```python
from build123d import *

# Parameters (mm, degrees)
BOSS_EXTRUDE1_DEPTH = 4


with BuildPart() as part:
    # Sketch1 → Boss-Extrude1 (new body)
    with BuildSketch(Plane.XY):
        with BuildLine():
            Line((6.07568334, -11), (11.008857545, -11))
            Line((11.008857545, -11), (11.008857545, 0))
            ThreePointArc((11.008857545, 0), (9.544391451, 3.535533906), (6.008857545, 5))
            Line((6.008857545, 5), (-5.92431666, 5))
            Line((-5.92431666, 5), (-5.92431666, -11))
            Line((-5.92431666, -11), (-1.92431666, -11))
            Line((-1.92431666, -11), (-1.92431666, -15))
            Line((-1.92431666, -15), (6.07568334, -15))
            Line((6.07568334, -15), (6.07568334, -11))
        make_face()
    extrude(amount=BOSS_EXTRUDE1_DEPTH)


solid = part.part
```
The model under review builds one solid part; all positions refer to its coordinate system, in mm. A direction names the side the tool comes from. Coordinates: 2 decimals unless noted, no trailing zeros. Write each loop counter-clockwise with the first axis right and the second up, starting at its lowest first coordinate (ties: lowest second). Pieces come first, ordered by that corner, then holes.
1) We need section A-A on z = 2.2. State the section outline as (x, y) points.
2) To check wall thickness, follow probe 1 along X at (y, z) = (-12.25, 2.2); probe 2 along Y at (x, z) = (-2, 2.45); probe 3 along X at (y, z) = (0.25, 1.1). State the ranges of each line that lie inside material, in increasing order.
3) We need section B-B on x = -3.25. State the section outline as (y, z) points.
4) Machinability: for faces 1 (the face through (-1.924, -13, 2)), 2 (the face through (6.076, -13, 2)), 3 (the face through (2, -5, 4)), which of the approach directions +Z, -Z, +X, -X, +Y, -Y give a long, thin tool a straight path to every point of the face, cutting with its end or side? Answer none if there is none.
5) We need section C-C on y = 2.5. State the section outline as (x, z) points, then the cut area to 3 significant figures.
6) Clearance check with flat-ended pins moving along their axes: pin 1 Ø1 at (x, z) = (7.5, 1.5) entering from +Y; pin 2 Ø2 at (x, z) = (-5, 1) entering from -Y. State where each tip first meets the part, or that it passes through.
Answer list:
1. outline: (-5.92, -11) - (-1.92, -11) - (-1.92, -15) - (6.08, -15) - (6.08, -11) - (11.01, -11) - (11.01, 0) arc R5 ccw to (6.01, 5) - (-5.92, 5) - close
2. probe 1: x = -1.92 to 6.08
2. probe 2: y = -11 to 5
2. probe 3: x = -5.92 to 11
3. outline: (-11, 0) - (5, 0) - (5, 4) - (-11, 4) - close
4. face 1: +Z, -Z, -X, -Y
4. face 2: +Z, -Z, +X, -Y
4. face 3: +Z, +X, -X, +Y, -Y
5. outline: (-5.92, 0) - (10.34, 0) - (10.34, 4) - (-5.92, 4) - close
5. area: 65.1 mm2
6. pin 1: stops at y = 4.9
6. pin 2: stops at y = -11
